from build123d import *

# Parameters (mm, degrees)
SKETCH1_W           = 100
SKETCH1_H           = 100
BOSS_EXTRUDE1_DEPTH = 100
SKETCH2_R           = 25
CUT_EXTRUDE1_DEPTH  = 30
CUT_EXTRUDE2_DEPTH  = 20


with BuildPart() as part:
    # Sketch1 → Boss-Extrude1 (new body)
    with BuildSketch(Plane(origin=(0, 0, 0), x_dir=(1, 0, 0), z_dir=(0, 1, 0))):
        Rectangle(SKETCH1_W, SKETCH1_H)
    extrude(amount=BOSS_EXTRUDE1_DEPTH)

    # Sketch2 → Cut-Extrude1 (cut)
    with BuildSketch(Plane.XY.offset(50)):
        with Locations((0, 50)):
            Circle(SKETCH2_R)
    extrude(amount=-CUT_EXTRUDE1_DEPTH, mode=Mode.SUBTRACT)

    # Sketch3 → Cut-Extrude2 (cut)
    with BuildSketch(Plane(origin=(0, 100, 0), x_dir=(1, 0, 0), z_dir=(0, 1, 0))):
        Polygon((0, 34.641016151), (-30, -17.320508076), (30, -17.320508076), align=None)
    extrude(amount=-CUT_EXTRUDE2_DEPTH, mode=Mode.SUBTRACT)


solid = part.part
Geometry check sheet. Reference: the model listing, model coordinates, mm. A direction names the side the tool comes from. Give positions to 0.01 mm unless a question says otherwise; leave off trailing zeros. Write each loop counter-clockwise with the first axis right and the second up, starting at its lowest first coordinate (ties: lowest second). Pieces come first, ordered by that corner, then holes.
1) Set-up check for faces 1 (the face through (-1, 49, -50)), 2 (the face through (0, 80, -3)), 3 (the face through (-5.42, 25.594, 35.21)): record each of +Z, -Z, +X, -X, +Y, -Y from which the full face is reachable in a straight line by a thin tool's end or side.
Values follow:
face 1: -Z, +X, -X, +Y, -Y
face 2: +Y
face 3: +Z
2) Thickness scan on line 1 (Y direction, x = 0, z = 32); line 2 (Y direction, x = -3.5, z = -1); line 3 (Z direction, x = -27, y = 94). Record the ranges inside material, lowest first.
Values follow:
line 1: y = 0 to 25, 75 to 100
line 2: y = 0 to 80
line 3: z = -50 to 12.12, 17.32 to 50
3) Cross-section at D-D (x = 21). Record the boundary of the cut face in (y, z), plus the area to 3 significant figures.
Values follow:
outline: (0, -50) - (100, -50) - (100, 1.73) - (80, 1.73) - (80, 17.32) - (100, 17.32) - (100, 50) - (63.56, 50) - (63.56, 20) - (36.44, 20) - (36.44, 50) - (0, 50) - close
area: 8,870 mm2
4) Go/stop test with a flat-tipped pin: pin 1 Ø6 at (x, y) = (-20, 46.5) entering from +Z. Record where the tip stops, or that it passes through.
Values follow:
pin 1: stops at z = 20
5) Cross-section at A-A (y = 87.5). Record the boundary of the cut face in (x, z), plus the area to 3 significant figures.
Values follow:
outline: (-50, -50) - (50, -50) - (50, 50) - (-50, 50) - close; hole (-30, 17.32) - (0, -34.64) - (30, 17.32) - close
area: 8,440 mm2
6) Cross-section at B-B (z = 30). Record the boundary of the cut face in (x, y).
Values follow:
outline: (-50, 0) - (50, 0) - (50, 100) - (-50, 100) - close; hole circle Ø50 at (0, 50)
7) Release check for a two-part mould opening along X. For faces 4 (the face through (-50, 49, 1)), 5 (the face through (-12, 27, 50)), 6 (the face through (0, 90, 17.321)), 7 (the face through (-14.79, 90.14, -9.02)) record: released by +X, released by -X, zero draft, split by the parting line, or undercut.
Values follow:
face 4: released by -X
face 5: zero draft
face 6: undercut
face 7: undercut
8) Cross-section at C-C (y = 50). Record the boundary of the cut face in (x, z), plus the area to 3 significant figures.
Values follow:
outline: (-50, -50) - (50, -50) - (50, 50) - (25, 50) - (25, 20) - (-25, 20) - (-25, 50) - (-50, 50) - close
area: 8,500 mm2
